from build123d import *

# Parameters (mm, degrees)
F0_W     = 228.6
F0_H     = 419.1
F1_DEPTH = 6.35
F2_W     = 76.708
F2_H     = 76.708
F3_DEPTH = 25.4
F4_R     = 38.1
F5_DEPTH = 25.4


with BuildPart() as f1:
    # F0 (on Top) → F1 (new body)
    with BuildSketch(Plane.XY):
        with Locations((16.350647, 15.597903)):
            Rectangle(F0_W, F0_H)
    extrude(amount=F1_DEPTH)

    # F2 (on face) → F3 (cut)
    with BuildSketch(Plane(origin=(0, 0, 0), x_dir=(1, 0, 0), z_dir=(0, 0, -1))):
        with Locations((-40.545353, 136.548097)):
            Rectangle(F2_W, F2_H)
        with Locations((-40.545353, 34.948097)):
            Rectangle(F2_W, F2_H)
        with Locations((-40.545353, -66.651903)):
            Rectangle(F2_W, F2_H)
        with Locations((-40.545353, -168.251903)):
            Rectangle(F2_W, F2_H)
    extrude(amount=-F3_DEPTH, mode=Mode.SUBTRACT)

    # F4 (on face) → F5 (cut)
    with BuildSketch(Plane(origin=(0, 0, 0), x_dir=(1, 0, 0), z_dir=(0, 0, -1))):
        with Locations((73.500647, 136.802097)):
            Circle(F4_R)
        with Locations((73.500647, 35.202097)):
            Circle(F4_R)
        with Locations((73.500647, -66.397903)):
            Circle(F4_R)
        with Locations((73.500647, -167.997903)):
            Circle(F4_R)
    extrude(amount=-F5_DEPTH, mode=Mode.SUBTRACT)


solid = f1.part
Geometry check sheet. Reference: the model listing, model coordinates, mm. Round coordinates to 2 decimals unless told otherwise and drop trailing zeros. Loops run counter-clockwise (first coordinate to the right, second up) from the corner with the lowest first, then second, coordinate; pieces in that order, holes last. Notation, with made-up numbers: (33.25, -0.5) - (68.25, -0.5) arc R12 ccw to (68.25, 20.5) - close; hole circle Ø3 at (-25.5, -38.75). An arc over 180 degrees is marked (long way). Answer as CSV lines item,"result".
(1) Material ranges on line 1 along Y through (x, z) = (-44, 1); line 2 along X through (y, z) = (-39.5, 5); line 3 along X through (y, z) = (-131.5, 2.75), recorded low to high.
Output values:
line 1,"y = -193.95 to -174.9, -98.19 to -73.3, 3.41 to 28.3, 105.01 to 129.9, 206.61 to 225.15"
line 2,"x = -97.95 to -78.9, -2.19 to 35.64, 111.36 to 130.65"
line 3,"x = -97.95 to -78.9, -2.19 to 35.77, 111.23 to 130.65"
(2) Cross-section at D-D, the plane y = -160. Enter the section's corners in (x, z).
Output values:
outline,"(-97.95, 0) - (-78.9, 0) - (-78.9, 6.35) - (-97.95, 6.35) - close; (-2.19, 0) - (43.28, 0) - (43.28, 6.35) - (-2.19, 6.35) - close; (103.72, 0) - (130.65, 0) - (130.65, 6.35) - (103.72, 6.35) - close"
(3) Release check for a two-part mould opening along Y. For faces 1 (the face through (68.541, -174.578, 3.131)), 2 (the face through (15, 19, 0)) record: released by +Y, released by -Y, zero draft, split by the parting line, or undercut.
Output values:
face 1,"undercut"
face 2,"zero draft"
(4) Cross-section at A-A, the plane x = -33. Enter the section's corners in (y, z), and give its area (3 significant figures).
Output values:
outline,"(-193.95, 0) - (-174.9, 0) - (-174.9, 6.35) - (-193.95, 6.35) - close; (-98.19, 0) - (-73.3, 0) - (-73.3, 6.35) - (-98.19, 6.35) - close; (3.41, 0) - (28.3, 0) - (28.3, 6.35) - (3.41, 6.35) - close; (105.01, 0) - (129.9, 0) - (129.9, 6.35) - (105.01, 6.35) - close; (206.61, 0) - (225.15, 0) - (225.15, 6.35) - (206.61, 6.35) - close"
area,"713 mm²"
(5) Cross-section at C-C, the plane z = 3. Give the number of separate pieces and of enclosed holes in the cut face, and give its area (3 significant figures).
Output values:
separate pieces,"1"
enclosed holes,"8"
area,"54,000 mm²"
(6) Cross-section at B-B, the plane y = 42. Enter the section's corners in (x, z).
Output values:
outline,"(-97.95, 0) - (-78.9, 0) - (-78.9, 6.35) - (-97.95, 6.35) - close; (-2.19, 0) - (44.24, 0) - (44.24, 6.35) - (-2.19, 6.35) - close; (102.76, 0) - (130.65, 0) - (130.65, 6.35) - (102.76, 6.35) - close"
